Here's how the part is built. I have some questions about the finished solid (model axes, mm). A direction names the side the tool comes from. Give positions to 0.01 mm unless a question says otherwise; leave off trailing zeros. Loops run counter-clockwise (first coordinate to the right, second up) from the corner with the lowest first, then second, coordinate; pieces in that order, holes last. Notation, with made-up numbers: (22, 74.25) - (59, 74.25) arc R35 ccw to (59, 110.25) - close; hole circle Ø9 at (0, 67.5). An arc over 180 degrees is marked (long way). Use one line per item in the form item = value.
from build123d import *

# Parameters (mm, degrees)
F1_DEPTH = 63.5
F0_W     = 25.4
F0_H     = 19.0500033191
F2_DEPTH = 50.8
F3_DEPTH = 15.875


# Not quite as in the source:
# - ends of sketch curves that miss each other by under 0.0002 mm in the source are joined


with BuildPart() as f1:
    # F0 (on Front) → F1 (new body, symmetric)
    with BuildSketch(Plane.XZ):
        Polygon((-41.275, 9.525), (-41.275, -9.525), (41.275, -9.525), (41.275, 9.525), (22.225, 9.525), align=None)
    extrude(amount=F1_DEPTH, both=True)

    # F0 (on Front) → F2 (join)
    with BuildSketch(Plane.XZ):
        with BuildLine():
            Line((22.225, 9.525), (41.275, 9.525))
            Line((41.275, 9.525), (41.275, 27.0002))
            ThreePointArc((41.275, 27.0002), (45.9246798487, 38.2255201513), (57.15, 42.8752))
            Line((57.15, 42.8752), (60.325, 42.8751966809))
            Line((60.325, 42.8751966809), (60.325, 61.9252))
            Line((60.325, 61.9252), (57.15, 61.9252))
            add(Edge.make_bspline(
                [(56.1392549791, 61.9105712312), (56.4777228602, 61.916713038), (56.8146554612, 61.9215892093), (57.15, 61.9252)],
                knots=[110.5401994714, 110.5401994714, 110.5401994714, 110.5401994714, 111.5045361635, 111.5045361635, 111.5045361635, 111.5045361635], degree=3))
            ThreePointArc((56.1392549791, 61.9105712312), (32.0994920725, 51.3359284167), (22.225, 27.0002))
            Line((22.225, 27.0002), (22.225, 9.525))
        make_face()
        with Locations((73.025, 52.4001983404)):
            Rectangle(F0_W, F0_H)
    extrude(amount=F2_DEPTH)

    # F0 (on Front) → F3 (join)
    with BuildSketch(Plane.XZ):
        with BuildLine():
            add(Edge.make_bspline(
                [(-41.275, 9.525), (-41.6296994967, 43.8725434099), (17.341283892, 61.2065468529), (56.1392549791, 61.9105712312)],
                knots=[0, 0, 0, 0, 110.5401994714, 110.5401994714, 110.5401994714, 110.5401994714], degree=3))
            Line((-41.275, 9.525), (22.225, 9.525))
            Line((22.225, 9.525), (22.225, 27.0002))
            ThreePointArc((22.225, 27.0002), (32.0994920725, 51.3359284167), (56.1392549791, 61.9105712312))
        make_face()
    extrude(amount=F3_DEPTH)


solid = f1.part
(1) If we section it at A-A (x = 65): List the corners of the cut face in (y, z) for me.
Geometry says:
outline = (-50.8, 42.88) - (0, 42.88) - (0, 61.93) - (-50.8, 61.93) - close
(2) For faces 1 (the flat face through (41.275, -1, 4)), 2 (the flat face through (1, 31, 9.525)), 3 (the flat face through (22.225, -33, 18)), 4 (the flat face through (46, -50.8, 42)), which set-ups out of +Z, -Z, +X, -X, +Y, -Y let a thin tool reach every point of the face, with its end or its side?
Geometry says:
face_1 = -Z, +X, +Y, -Y
face_2 = +Z, +X, -X, +Y
face_3 = +Z, -X, -Y
face_4 = +Z, +X, -X, -Y
(3) If we section it at B-B (y = 29): List the corners of the cut face in (x, z) for me (3 decimals).
Geometry says:
outline = (-41.275, -9.525) - (41.275, -9.525) - (41.275, 9.525) - (-41.275, 9.525) - close
(4) If I drill on probe 1 along Z at (x, y) = (-16, 11.5) (3 decimals); probe 2 along X at (y, z) = (-19.5, 25) (3 decimals); probe 3 along Y at (x, z) = (2, 24) (3 decimals), over which ranges is the centre line in solid material (lowest first)?
Geometry says:
probe_1 = -9.525 to 9.525
probe_2 = 22.225 to 41.275
probe_3 = -15.875 to 0
(5) For P1, Ø5, axis at y = -33, z = 15, coming from the -X side (3 decimals); P2, Ø1, axis at x = 59.5, y = -25.5, coming from the -Z side; P3, Ø2, axis at x = 44, z = 38.5, coming from the -Y side, each with a flat end and sliding along its axis, tell me the tip position at first contact or that it passes through.
Geometry says:
P1 = 22.225
P2 = 42.88
P3 = -50.8
